The listing builds one solid part. Answer for the finished solid, in the listing's coordinates (mm). Round coordinates to 2 decimals unless told otherwise and drop trailing zeros. Write each loop counter-clockwise with the first axis right and the second up, starting at its lowest first coordinate (ties: lowest second). Pieces come first, ordered by that corner, then holes.
Item 1: Find section A-A on z = 51.5. Give the vertices of the cut face in (x, y), then the cut area to 3 significant figures.
Item 2: Find section C-C on y = -31.5. Give the vertices of the cut face in (x, z), then the cut area to 3 significant figures.
Item 3: Find the intervals of material crossed by probe 1 along Y at (x, z) = (-1.5, 13.5); probe 2 along Z at (x, y) = (-0.5, -36); probe 3 along Z at (x, y) = (-3.25, -41), in increasing order.
Item 4: Find section B-B on x = -3.75. Give the vertices of the cut face in (y, z), then the cut area to 3 significant figures.
Item 5: Each of these flat-tipped pins is pushed along its axis until it touches: pin 1 (3 mm diameter, centred on x = 1, y = -41, fed in from -Z); pin 2 (4 mm diameter, centred on x = -2, y = -38.5, fed in from +Z); pin 3 (12 mm diameter, centred on y = -3.5, z = 98, fed in from +X); pin 4 (2 mm diameter, centred on x = -3, y = -34.5, fed in from +Z). Where does it stop, or does it pass through?
```python
from build123d import *

# Parameters (mm, degrees)
SKETCH1_W           = 2.54
SKETCH1_H           = 2.54
BOSS_EXTRUDE1_DEPTH = 111.76
SKETCH2_W           = 2.54
SKETCH2_H           = 2.54
BOSS_EXTRUDE2_DEPTH = 40.64
SKETCH3_W           = 2.54
SKETCH3_H           = 2.54
BOSS_EXTRUDE3_DEPTH = 111.76
SKETCH5_W           = 2.54
SKETCH5_H           = 2.54
BOSS_EXTRUDE4_DEPTH = 2.54
SKETCH6_W           = 2.54
SKETCH6_H           = 2.54
BOSS_EXTRUDE5_DEPTH = 2.54
SKETCH7_W           = 2.54
SKETCH7_H           = 2.54
BOSS_EXTRUDE6_DEPTH = 1.27


with BuildPart() as part:
    # Sketch1 → Boss-Extrude1 (new body)
    with BuildSketch(Plane.XY):
        with Locations((-1.27, 1.27)):
            Rectangle(SKETCH1_W, SKETCH1_H)
    extrude(amount=BOSS_EXTRUDE1_DEPTH)

    # Sketch2 → Boss-Extrude2 (add)
    with BuildSketch(Plane.XZ):
        with Locations((-1.27, 1.27)):
            Rectangle(SKETCH2_W, SKETCH2_H)
    extrude(amount=BOSS_EXTRUDE2_DEPTH)

    # Sketch3 → Boss-Extrude3 (add)
    with BuildSketch(Plane(origin=(0, 0, 0), x_dir=(-1, 0, 0), z_dir=(0, 0, -1))):
        with Locations((1.27, -41.91)):
            Rectangle(SKETCH3_W, SKETCH3_H)
    extrude(amount=-BOSS_EXTRUDE3_DEPTH)

    # Sketch5 → Boss-Extrude4 (add)
    with BuildSketch(Plane.ZY.offset(2.54)):
        with Locations((107.95, 1.27)):
            Rectangle(SKETCH5_W, SKETCH5_H)
    boss_extrude4 = extrude(amount=BOSS_EXTRUDE4_DEPTH)

    # Sketch6 → Boss-Extrude5 (add)
    with BuildSketch(Plane(origin=(0, 0, 0), x_dir=(0, 0, -1), z_dir=(1, 0, 0))):
        with Locations((-107.95, 1.27)):
            Rectangle(SKETCH6_W, SKETCH6_H)
    boss_extrude5 = extrude(amount=BOSS_EXTRUDE5_DEPTH)

    # Sketch7 → Boss-Extrude6 (add)
    with BuildSketch(Plane(origin=(0, 0, 0), x_dir=(-1, 0, 0), z_dir=(0, -1, 0))):
        with Locations((3.81, -107.95)):
            Rectangle(SKETCH7_W, SKETCH7_H)
        with Locations((-1.27, -107.95)):
            Rectangle(SKETCH7_W, SKETCH7_H)
    boss_extrude6 = extrude(amount=BOSS_EXTRUDE6_DEPTH)

    # Mirror1: Boss-Extrude4, Boss-Extrude5, Boss-Extrude6 across plane
    add(boss_extrude4.mirror(Plane(origin=(0, -20.32, 0), x_dir=(0, 0, 1), z_dir=(0, -1, 0))))
    add(boss_extrude5.mirror(Plane(origin=(0, -20.32, 0), x_dir=(0, 0, 1), z_dir=(0, -1, 0))))
    add(boss_extrude6.mirror(Plane(origin=(0, -20.32, 0), x_dir=(0, 0, 1), z_dir=(0, -1, 0))))


solid = part.part
```
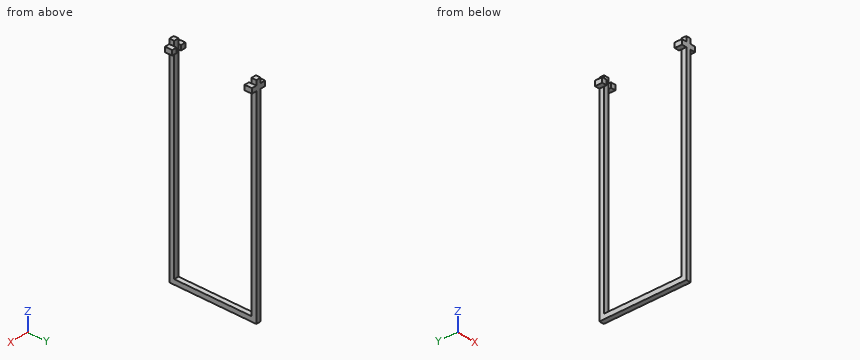
Check values:
1. outline: (-2.54, -43.18) - (0, -43.18) - (0, -40.64) - (-2.54, -40.64) - close; (-2.54, 0) - (0, 0) - (0, 2.54) - (-2.54, 2.54) - close
1. area: 12.9 mm2
2. outline: (-2.54, 0) - (0, 0) - (0, 2.54) - (-2.54, 2.54) - close
2. area: 6.45 mm2
3. probe 1: y = -43.18 to -40.64, 0 to 2.54
3. probe 2: z = 0 to 2.54
3. probe 3: z = 106.68 to 109.22
4. outline: (-43.18, 106.68) - (-39.37, 106.68) - (-39.37, 109.22) - (-43.18, 109.22) - close; (-1.27, 106.68) - (2.54, 106.68) - (2.54, 109.22) - (-1.27, 109.22) - close
4. area: 19.4 mm2
5. pin 1: stops at z = 0
5. pin 2: stops at z = 109.22
5. pin 3: stops at x = 0
5. pin 4: stops at z = 2.54
